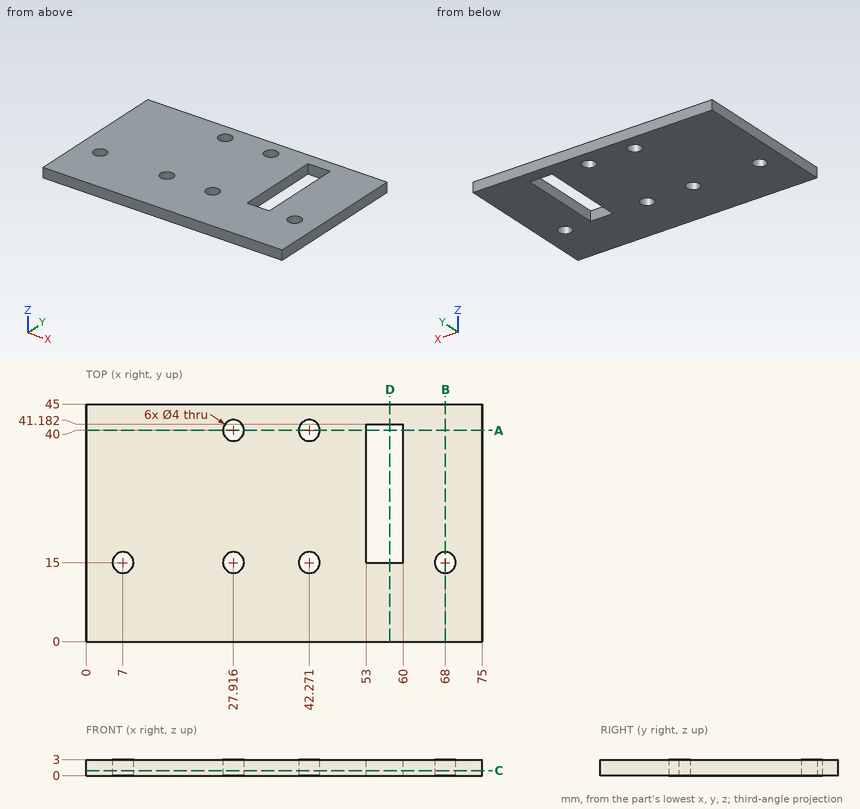
Study the drawing (mm; zero at the part's minimum x, y, z) and answer. Round coordinates to 2 decimals unless told otherwise and drop trailing zeros. Order: outer loops, then holes, each group sorted by start corner. A loop starts at its lowest first (then second) coordinate and runs counter-clockwise, first axis right, second up. Notation, with made-up numbers: (86.25, 48) - (107.25, 48) arc R34 ccw to (107.25, 82) - close; hole circle Ø6 at (-15.5, 1.25). An arc over 180 degrees is marked (long way). Use one line per item in the form item = value. Start each with the question number.
(1) The part is cut by section B-B (x = 68). Give the vertices of the cut face in (y, z), then the cut area to 3 significant figures.
(2) The part is cut by section C-C (z = 0.95). Give the vertices of the cut face in (x, y), then the cut area to 3 significant figures.
(3) The part is cut by section A-A (y = 40). Give the vertices of the cut face in (x, z), then the cut area to 3 significant figures.
(4) The part is cut by section D-D (x = 57.5). Give the vertices of the cut face in (y, z).
(5) Find the intervals of material crossed by line 1 along X through (y, z) = (34.5, 2.2); line 2 along Y through (x, z) = (29, 2); line 3 along X through (y, z) = (38.5, 2.2) (1 decimal), in increasing order. Write a range as from..to.
Checked values:
q1.outline = (0, 0) - (13, 0) - (13, 3) - (0, 3) - close; (17, 0) - (45, 0) - (45, 3) - (17, 3) - close
q1.area = 123 mm^2
q2.outline = (0, 0) - (75, 0) - (75, 45) - (0, 45) - close; hole circle Ø4 at (7, 15); hole circle Ø4 at (27.92, 15); hole circle Ø4 at (27.92, 40); hole circle Ø4 at (42.27, 15); hole circle Ø4 at (42.27, 40); hole (53, 15) - (60, 15) - (60, 41.18) - (53, 41.18) - close; hole circle Ø4 at (68, 15)
q2.area = 3,120 mm^2
q3.outline = (0, 0) - (25.92, 0) - (25.92, 3) - (0, 3) - close; (29.92, 0) - (40.27, 0) - (40.27, 3) - (29.92, 3) - close; (44.27, 0) - (53, 0) - (53, 3) - (44.27, 3) - close; (60, 0) - (75, 0) - (75, 3) - (60, 3) - close
q3.area = 180 mm^2
q4.outline = (0, 0) - (15, 0) - (15, 3) - (0, 3) - close; (41.18, 0) - (45, 0) - (45, 3) - (41.18, 3) - close
q5.line_1 = 0..53, 60..75
q5.line_2 = 0..13.32, 16.68..38.32, 41.68..45
q5.line_3 = 0..26.6, 29.2..40.9, 43.6..53, 60..75
